CAD build for the part. Positions are in the model's coordinates, mm. A direction names the side the tool comes from. Round coordinates to 2 decimals unless told otherwise and drop trailing zeros. Order: outer loops, then holes, each group sorted by start corner. A loop starts at its lowest first (then second) coordinate and runs counter-clockwise, first axis right, second up. Notation, with made-up numbers: (-8, 11) -> (12, 11) arc R8 ccw to (12, 15) -> close; hole circle Ø6 at (60.5, -36). An arc over 180 degrees is marked (long way). Return JSON: item names as keys, results as strings. Group by question number.
Q1. Probe line 1 along Y through (x, z) = (-22, -4.5); line 2 along Y through (x, z) = (9.5, -58.5); line 3 along Z through (x, y) = (7, 1.5). List the from-to ranges inside material, lowest first.
Q2. Cut at C-C (z = 8). Write the cut outline in (x, y).
Q3. Cut at A-A (y = -9.5). Write the cut outline in (x, z).
Q4. Mould opens along Z. For faces 1 (the flat face through (29.447, -9.93, -22.105)), 2 (the flat face through (-33.434, 14.93, -34.376)), 3 (the cylindrical face through (-27.223, -9.93, -30.007)) say: +Z half, -Z half, draft (parallel to the pull), parting line (faces both ways), or undercut.
Q5. Cut at D-D (x = 23). Write the cut outline in (y, z).
Q6. Cut at B-B (x = 0). Write the cut outline in (y, z).
Q7. Which spindle directions (+Z, -Z, +X, -X, +Y, -Y) get a long thin tool onto all of the face, cutting with end or side? Do faces 4 (the flat face through (-33.434, -9.93, -34.376)), 5 (the cylindrical face through (-0.377, 14.93, -9.955)), 6 (the flat face through (-1, 15, 0.044)), 7 (the cylindrical face through (17.06, -9.93, -61.29)). Say none if no direction does.
Q8. Flat gauge pins, fed straight in: pin 1 (10 mm diameter, centred on x = 41.5, y = 9, fed in from +Z); pin 2 (1.5 mm diameter, centred on y = 8, z = -42.5, fed in from +X); pin 3 (11 mm diameter, centred on x = -2.5, y = 16.5, fed in from +Z); pin 4 (3 mm diameter, centred on y = -7.5, z = -52, fed in from -X). Where does each tip first touch, or does it go through?
from build123d import *

# Parameters (mm, degrees)
BOSS_EXTRUDE1_START  = -15
BOSS_EXTRUDE1_DEPTH  = 15
BOSS_EXTRUDE2_DEPTH  = 10
CIRPATTERN1_COUNT    = 5
MIRROR3_COPY_1_DEPTH = 10
MIRROR3_COPY_2_DEPTH = 10
MIRROR3_COPY_3_DEPTH = 10
MIRROR3_COPY_4_DEPTH = 10


with BuildPart() as part:
    # Sketch1 → Revolve1 (revolve)
    with BuildSketch(Plane.YZ, mode=Mode.PRIVATE) as revolve1_sk:
        Polygon((-4.999994159, -22.251027603), (-4.999994159, 15.415581909), (5.841e-06, 15.415581909), (5.841e-06, 0.109652172), (5.000005841, 0.109652172), (5.000005841, 15.109652172), (10.000005841, 15.109652172), (10.000005841, 0.109652172), (10.000005841, -25.956139131), (-4.999994159, -25.956139131), align=None)
    revolve(revolve1_sk.sketch.rotate(Axis((0, -19.999999988, -38.456139131), (0, 1, 0)), 180), axis=Axis((0, -19.999999988, -38.456139131), (0, 1, 0)))

    # Sketch2 → Boss-Extrude1 (add)
    with BuildSketch(Plane(origin=(0, 10.000005841, 0), x_dir=(1, 0, 0), z_dir=(0, 1, 0)).offset(BOSS_EXTRUDE1_START)):
        with BuildLine():
            Line((-2.5, 31.208690417), (2.5, 31.208690417))
            Line((2.5, 31.208690417), (2.5, 26.208690417))
            ThreePointArc((2.5, 26.208690417), (0, 25.956139131), (-2.5, 26.208690417))
            Line((-2.5, 26.208690417), (-2.5, 31.208690417))
        make_face()
    extrude(amount=BOSS_EXTRUDE1_DEPTH)

    # Sketch3 → Boss-Extrude2 (add)
    with BuildSketch(Plane.XZ.offset(4.999994159)):
        with BuildLine():
            Line((-6.45112782, 0.043860869), (5.54887218, 0.043860869))
            Line((5.54887218, 0.043860869), (5.54887218, -10.496030583))
            ThreePointArc((5.54887218, -10.496030583), (-0.461398285, -9.956302999), (-6.45112782, -10.689649467))
            Line((-6.45112782, -10.689649467), (-6.45112782, 0.043860869))
        make_face()
    boss_extrude2 = extrude(amount=BOSS_EXTRUDE2_DEPTH)

    # CirPattern1: Boss-Extrude2 ×5 about axis
    cirpattern1_axis = Axis((0, 0, -38.456139131), (0, 1, 0))
    for i in range(1, CIRPATTERN1_COUNT):
        add(boss_extrude2.rotate(cirpattern1_axis, i * 360 / CIRPATTERN1_COUNT))

    # Mirror3: Boss-Extrude2 across plane
    add(boss_extrude2.mirror(Plane(origin=(0, 2.500005841, 0), x_dir=(0, 0, 1), z_dir=(0, -1, 0))))

    # Mirror3 copy 1 sketch → Mirror3 copy 1 (add)
    with BuildSketch(Plane(origin=(36.573961712, 10.000005841, -26.572538602), x_dir=(0.30901699437494745, 4.31570827698209e-15, -0.9510565162951535), z_dir=(0, 1, 0))):
        with BuildLine():
            Line((-6.45112782, -0.043860869), (5.54887218, -0.043860869))
            Line((5.54887218, -0.043860869), (5.54887218, 10.496030583))
            ThreePointArc((5.54887218, 10.496030583), (-0.461398285, 9.956302999), (-6.45112782, 10.689649467))
            Line((-6.45112782, 10.689649467), (-6.45112782, -0.043860869))
        make_face()
    extrude(amount=MIRROR3_COPY_1_DEPTH)

    # Mirror3 copy 2 sketch → Mirror3 copy 2 (add)
    with BuildSketch(Plane(origin=(22.603951441, 10.000005841, -69.567809226), x_dir=(-0.8090169943749473, -1.1298670954668355e-14, -0.5877852522924732), z_dir=(0, 1, 0))):
        with BuildLine():
            Line((-6.45112782, -0.043860869), (5.54887218, -0.043860869))
            Line((5.54887218, -0.043860869), (5.54887218, 10.496030583))
            ThreePointArc((5.54887218, 10.496030583), (-0.461398285, 9.956302999), (-6.45112782, 10.689649467))
            Line((-6.45112782, 10.689649467), (-6.45112782, -0.043860869))
        make_face()
    extrude(amount=MIRROR3_COPY_2_DEPTH)

    # Mirror3 copy 3 sketch → Mirror3 copy 3 (add)
    with BuildSketch(Plane(origin=(-22.603951441, 10.000005841, -69.567809226), x_dir=(-0.8090169943749476, -1.1298670954668358e-14, 0.587785252292473), z_dir=(0, 1, 0))):
        with BuildLine():
            Line((-6.45112782, -0.043860869), (5.54887218, -0.043860869))
            Line((5.54887218, -0.043860869), (5.54887218, 10.496030583))
            ThreePointArc((5.54887218, 10.496030583), (-0.461398285, 9.956302999), (-6.45112782, 10.689649467))
            Line((-6.45112782, 10.689649467), (-6.45112782, -0.043860869))
        make_face()
    extrude(amount=MIRROR3_COPY_3_DEPTH)

    # Mirror3 copy 4 sketch → Mirror3 copy 4 (add)
    with BuildSketch(Plane(origin=(-36.573961712, 10.000005841, -26.572538602), x_dir=(0.30901699437494723, 4.315708276982087e-15, 0.9510565162951536), z_dir=(0, 1, 0))):
        with BuildLine():
            Line((-6.45112782, -0.043860869), (5.54887218, -0.043860869))
            Line((5.54887218, -0.043860869), (5.54887218, 10.496030583))
            ThreePointArc((5.54887218, 10.496030583), (-0.461398285, 9.956302999), (-6.45112782, 10.689649467))
            Line((-6.45112782, 10.689649467), (-6.45112782, -0.043860869))
        make_face()
    extrude(amount=MIRROR3_COPY_4_DEPTH)


solid = part.part
Solution:
{
 "1": {"line 1": "y = -5 to 0, 5 to 10", "line 2": "y = -5 to 10", "line 3": "z = -76.38 to -48.81, -28.1 to -0.53"},
 "2": {"outline": "(-27.28, -5) -> (27.28, -5) -> (27.28, 0) -> (-27.28, 0) -> close; (-26.67, 5) -> (26.67, 5) -> (26.67, 10) -> (-26.67, 10) -> close"},
 "3": {"outline": "(-38.61, -32.69) -> (-28.4, -36.01) arc R28.6 cw to (-24.88, -24.54) -> (-34.9, -21.28) -> close; (-27.12, -66.34) -> (-17.41, -73.4) -> (-11.1, -64.71) arc R28.6 cw to (-20.92, -57.81) -> close; (-6.45, -10.69) arc R28.6 cw to (5.55, -10.5) -> (5.55, 0.04) -> (-6.45, 0.04) -> close; (11.95, -64.34) -> (18.14, -72.86) -> (27.85, -65.81) -> (21.54, -57.13) arc R28.6 cw to start; (24.41, -23.74) arc R28.6 cw to (28.31, -35.09) -> (38.33, -31.84) -> (34.62, -20.42) -> close"},
 "4": {"face 1": "+Z half", "face 2": "-Z half", "face 3": "undercut"},
 "5": {"outline": "(-15, -69.33) -> (-5, -69.33) -> (-5, -87.17) -> (0, -87.17) -> (0, -69.41) -> (5, -69.41) -> (5, -86.83) -> (10, -86.83) -> (10, -69.33) -> (20, -69.33) -> (20, -59.14) -> (10, -59.14) -> (10, 9.92) -> (5, 9.92) -> (5, -7.5) -> (0, -7.5) -> (0, 10.26) -> (-5, 10.26) -> (-5, -59.14) -> (-15, -59.14) -> close"},
 "6": {"outline": "(-15, -9.95) -> (-5, -9.95) -> (-5, -31.21) -> (10, -31.21) -> (10, -9.95) -> (20, -9.95) -> (20, 0.04) -> (10, 0.04) -> (10, 15.11) -> (5, 15.11) -> (5, 0.11) -> (0, 0.11) -> (0, 15.42) -> (-5, 15.42) -> (-5, 0.04) -> (-15, 0.04) -> close; (-5, -92.33) -> (0, -92.33) -> (0, -77.02) -> (5, -77.02) -> (5, -92.02) -> (10, -92.02) -> (10, -50.96) -> (-5, -50.96) -> close"},
 "7": {"face 4": "-Z, -X, -Y", "face 5": "-Z, +Y", "face 6": "+Z, +X, -X, +Y", "face 7": "+Z, -Y"},
 "8": {"pin 1": "stops at z = 0.75", "pin 2": "stops at x = 53.46", "pin 3": "stops at z = 0.04", "pin 4": "passes through"}
}
